Job drawing, mm, ordinate dimensions from the low corner. One solid piece. Give positions to 0.01 mm unless a question says otherwise; leave off trailing zeros. Loops run counter-clockwise (first coordinate to the right, second up) from the corner with the lowest first, then second, coordinate; pieces in that order, holes last. Notation, with made-up numbers: (9.25, 57.25) - (17.25, 57.25) arc R10 cw to (17.25, 65.25) - close; hole circle Ø9 at (-15.75, 74). An arc over 180 degrees is marked (long way). Answer as CSV lines item,"result". Start each with the question number.
Item 1: Saw through at A-A on y = 57.15. Give the cut face in (x, z), plus the area to 3 significant figures.
Item 2: Pin check, flat tips, straight feed: pin 1 (5 mm diameter, centred on x = 59.5, z = 4.5, fed in from -Y); pin 2 (4 mm diameter, centred on x = 13, z = 4.5, fed in from -Y) (1 decimal); pin 3 (1 mm diameter, centred on x = 97, z = 11.5, fed in from -Y) (1 decimal). Stop position of each tip, or through.
Item 3: Drill centre lines: L1, parallel to Y at x = 30.5, z = 9.75 (1 decimal); L2, parallel to X at y = 47.5, z = 7.5 (1 decimal); L3, parallel to Y at x = 102, z = 4.5. Where is each one in solid material? Low to high. Write a range as from..to.
Item 4: Saw through at C-C on z = 2.25. Give the cut face in (x, y), plus the area to 3 significant figures.
Item 5: Pull direction Y, two halves, no side cores. Call the marked faces 1 and 2: pulls with the +Y half, pulls with the -Y half, needs draft (parallel to the pull), parting line crosses it, or undercut.
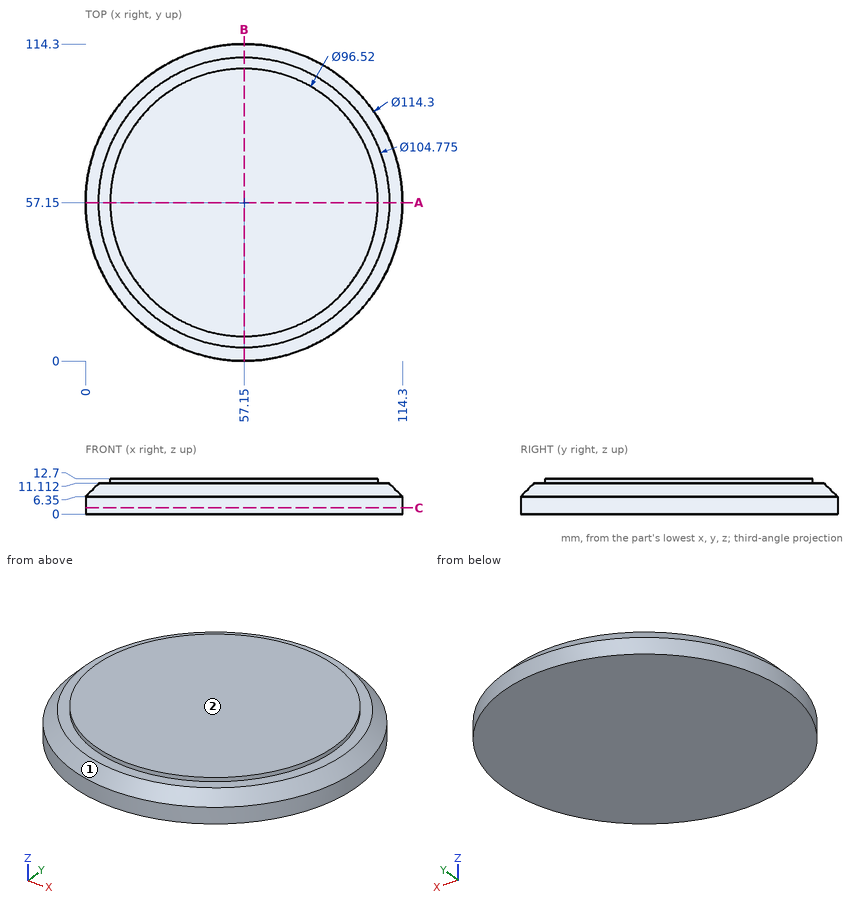
Responses:
1,outline,"(0, 0) - (114.3, 0) - (114.3, 6.35) - (109.54, 11.11) - (105.41, 11.11) - (105.41, 12.7) - (8.89, 12.7) - (8.89, 11.11) - (4.76, 11.11) - (0, 6.35) - close"
1,area,"1,400 mm2"
2,pin 1,"y = 0"
2,pin 2,"y = 18.6"
2,pin 3,"y = 22.8"
3,L1,"10.5..103.8"
3,L2,"2..112.3"
3,L3,"21.73..92.57"
4,outline,"circle Ø114.3 at (57.15, 57.15)"
4,area,"10,300 mm2"
5,face 1,"parting line crosses it"
5,face 2,"needs draft"
